The listing builds one solid part. Answer for the finished solid, in the listing's coordinates (mm). Face numbers are marked on the shaded views. A direction names the side the tool comes from. Coordinates: 2 decimals unless noted, no trailing zeros. Order: outer loops, then holes, each group sorted by start corner. A loop starts at its lowest first (then second) coordinate and runs counter-clockwise, first axis right, second up. Notation, with made-up numbers: (-21.5, 42.5) -> (37.5, 42.5) arc R27 ccw to (37.5, 61.5) -> close; hole circle Ø1 at (88.25, -29.75). An arc over 180 degrees is marked (long way). Return JSON: item names as keys, results as strings.
```python
from build123d import *

# Parameters (mm, degrees)
SKETCH_1_W          = 28
SKETCH_1_H          = 16
SKETCH_1_R          = 1.5
EXTRUDE_1_DEPTH     = 10
FILLET_1_R          = 3
SKETCH_2_R          = 1.5
EXTRUDE_2_DEPTH     = 0.4
CUT_EXTRUDE_1_DEPTH = 0.1
CUT_EXTRUDE_2_DEPTH = 3
CUT_EXTRUDE_3_DEPTH = 0.1
CUT_EXTRUDE_4_DEPTH = 0.1
SKETCH_7_W          = 2.9
SKETCH_7_H          = 0.1
CUT_EXTRUDE_5_DEPTH = 0.1
SKETCH_8_W          = 2.9
SKETCH_8_H          = 0.1
CUT_EXTRUDE_6_DEPTH = 0.1
EXTRUDE_3_DEPTH     = 4.5
SKETCH_11_W         = 10
SKETCH_11_H         = 0.8
EXTRUDE_4_DEPTH     = 6.5
SKETCH_12_R         = 0.75
CUT_EXTRUDE_7_DEPTH = 53.388166603
FILLET_2_R          = 1
SKETCH_13_R         = 0.75
CUT_EXTRUDE_8_DEPTH = 2


with BuildPart() as part:
    # Sketch 1 → Extrude 1 (new body)
    with BuildSketch(Plane(origin=(0, 0, 0), x_dir=(0, 0, -1), z_dir=(1, 0, 0))):
        Rectangle(SKETCH_1_W, SKETCH_1_H)
        with Locations((11, -5)):
            Circle(SKETCH_1_R, mode=Mode.SUBTRACT)
        with Locations((-11, 5)):
            Circle(SKETCH_1_R, mode=Mode.SUBTRACT)
    extrude(amount=EXTRUDE_1_DEPTH)

    # Fillet 1
    fillet_1_edges = [part.edges().sort_by_distance(p)[0] for p in [
        (5, 8, 14),
        (5, 8, -14),
        (5, -8, -14),
        (5, -8, 14),
    ]]
    fillet(fillet_1_edges, radius=FILLET_1_R)

    # Sketch 2 → Extrude 2 (add)
    # profile 1 of 2: a face of its own
    with BuildSketch(Plane(origin=(10, 0, 0), x_dir=(0, 0, -1), z_dir=(1, 0, 0))):
        with BuildLine():
            Line((13.5, -5), (13.5, -2.1))
            Line((13.5, -2.1), (11, -2.1))
            ThreePointArc((11, -2.1), (8.949390335, -2.949390335), (8.1, -5))
            Line((8.1, -5), (8.1, -7.5))
            Line((8.1, -7.5), (11, -7.5))
            ThreePointArc((11, -7.5), (12.767766953, -6.767766953), (13.5, -5))
        make_face()
        with Locations((11, -5)):
            Circle(SKETCH_2_R, mode=Mode.SUBTRACT)
    # profile 2 of 2: a face of its own
    with BuildSketch(Plane(origin=(10, 0, 0), x_dir=(0, 0, -1), z_dir=(1, 0, 0))):
        with BuildLine():
            Line((-11, 2.1), (-13.5, 2.1))
            Line((-13.5, 2.1), (-13.5, 5))
            ThreePointArc((-13.5, 5), (-12.767766953, 6.767766953), (-11, 7.5))
            Line((-11, 7.5), (-8.1, 7.5))
            Line((-8.1, 7.5), (-8.1, 5))
            ThreePointArc((-8.1, 5), (-8.949390335, 2.949390335), (-11, 2.1))
        make_face()
        with Locations((-11, 5)):
            Circle(SKETCH_2_R, mode=Mode.SUBTRACT)
    extrude(amount=EXTRUDE_2_DEPTH)

    # Sketch 3 → Cut-Extrude 1 (cut)
    with BuildSketch(Plane.ZY):
        with BuildLine():
            Line((-13.5, -2.1), (-11, -2.1))
            ThreePointArc((-11, -2.1), (-8.949390335, -2.949390335), (-8.1, -5))
            Line((-8.1, -5), (-8.1, -7.5))
            Line((-8.1, -7.5), (-8.1, -8))
            Line((-8.1, -8), (-8.2, -8))
            Line((-8.2, -8), (-8.2, -7.5))
            Line((-8.2, -7.5), (-8.2, -5))
            ThreePointArc((-8.2, -5), (-9.020101013, -3.020101013), (-11, -2.2))
            Line((-11, -2.2), (-13.5, -2.2))
            Line((-13.5, -2.2), (-14, -2.2))
            Line((-14, -2.2), (-14, -2.1))
            Line((-14, -2.1), (-13.5, -2.1))
        make_face()
        with BuildLine():
            Line((13.5, 2.1), (11, 2.1))
            ThreePointArc((11, 2.1), (8.949390335, 2.949390335), (8.1, 5))
            Line((8.1, 5), (8.1, 7.5))
            Line((8.1, 7.5), (8.1, 8))
            Line((8.1, 8), (8.2, 8))
            Line((8.2, 8), (8.2, 7.5))
            Line((8.2, 7.5), (8.2, 5))
            ThreePointArc((8.2, 5), (9.020101013, 3.020101013), (11, 2.2))
            Line((11, 2.2), (13.5, 2.2))
            Line((13.5, 2.2), (14, 2.2))
            Line((14, 2.2), (14, 2.1))
            Line((14, 2.1), (13.5, 2.1))
        make_face()
    extrude(amount=-CUT_EXTRUDE_1_DEPTH, mode=Mode.SUBTRACT)

    # Sketch 4 → Cut-Extrude 2 (cut)
    with BuildSketch(Plane(origin=(0, 8, 0), x_dir=(1, 0, 0), z_dir=(0, 1, 0))):
        Polygon((0, -8.2), (3.1, -8.2), (3.1, 14), (3, 14), (3, -8.1), (0, -8.1), align=None)
    extrude(amount=-CUT_EXTRUDE_2_DEPTH, mode=Mode.SUBTRACT)

    # Sketch 5 → Cut-Extrude 3 (cut)
    with BuildSketch(Plane(origin=(0, 0, -14), x_dir=(-1, 0, 0), z_dir=(0, 0, -1))):
        Polygon((-3, 5), (-3, -2.1), (-0.1, -2.1), (-0.1, -2.2), (-3.1, -2.2), (-3.1, 5), align=None)
    extrude(amount=-CUT_EXTRUDE_3_DEPTH, mode=Mode.SUBTRACT)

    # Sketch 6 → Cut-Extrude 4 (cut)
    with BuildSketch(Plane.ZY.offset(-3.1)):
        with BuildLine():
            Line((-8.2, -8), (11, -8))
            ThreePointArc((11, -8), (13.121320344, -7.121320344), (14, -5))
            Line((14, -5), (14, 2.1))
            Line((14, 2.1), (14, 2.2))
            Line((14, 2.2), (13.9, 2.2))
            Line((13.9, 2.2), (13.9, 2.1))
            Line((13.9, 2.1), (13.9, -5))
            ThreePointArc((13.9, -5), (13.050609665, -7.050609665), (11, -7.9))
            Line((11, -7.9), (-8.2, -7.9))
            Line((-8.2, -7.9), (-8.2, -8))
        make_face()
    extrude(amount=CUT_EXTRUDE_4_DEPTH, mode=Mode.SUBTRACT)

    # Sketch 7 → Cut-Extrude 5 (cut)
    with BuildSketch(Plane.XY.offset(14)):
        with Locations((1.55, 2.15)):
            Rectangle(SKETCH_7_W, SKETCH_7_H)
    extrude(amount=-CUT_EXTRUDE_5_DEPTH, mode=Mode.SUBTRACT)

    # Sketch 8 → Cut-Extrude 6 (cut)
    with BuildSketch(Plane.XZ.offset(8)):
        with Locations((1.55, -8.15)):
            Rectangle(SKETCH_8_W, SKETCH_8_H)
    extrude(amount=-CUT_EXTRUDE_6_DEPTH, mode=Mode.SUBTRACT)

    # Sketch 10 → Extrude 3 (add)
    with BuildSketch(Plane.ZY.offset(-3.1)):
        Polygon((-2.6, -8), (-2.6, -10), (49.4, -10), (49.4, -9.5), (-2.1, -9.5), (-2.1, -8), align=None)
        with BuildLine():
            Line((11, -8.08), (11, -8))
            Line((11, -8), (8.2, -8))
            Line((8.2, -8), (8.2, -8.08))
            ThreePointArc((8.2, -8.08), (9.6, -9.48), (11, -8.08))
        make_face()
    extrude(amount=-EXTRUDE_3_DEPTH)

    # Sketch 11 → Extrude 4 (add)
    with BuildSketch(Plane.ZY.offset(-2)):
        with Locations((-19, 3.6)):
            Rectangle(SKETCH_11_W, SKETCH_11_H)
        with Locations((-19, -2.2)):
            Rectangle(SKETCH_11_W, SKETCH_11_H)
        Polygon((-1, 8), (-1, 10.5), (-10.5, 10.5), (-10.5, 9.7), (-1.8, 9.7), (-1.8, 8), align=None)
    extrude(amount=-EXTRUDE_4_DEPTH)

    # Sketch 12 → Cut-Extrude 7 (cut, through all)
    with BuildSketch(Plane(origin=(0, 4, 0), x_dir=(1, 0, 0), z_dir=(0, 1, 0))):
        with Locations(Location((5.25, 20, 0), (0, 0, 270))):
            Circle(SKETCH_12_R)
        Polygon((2, 17.5), (3, 17.5), (3, 22), (4.154700538, 24), (3, 24), (2, 24), align=None)
        Polygon((8.5, 24), (8.5, 17.5), (7.5, 17.5), (7.5, 22), (6.345299462, 24), (7.5, 24), align=None)
    extrude(amount=-CUT_EXTRUDE_7_DEPTH, mode=Mode.SUBTRACT)

    # Fillet 2
    fillet_2_edges = [part.edges().sort_by_distance(p)[0] for p in [
        (5.35, -10, -2.6),
        (5.35, -9.5, -2.1),
        (5.25, 9.7, -1.8),
        (5.25, 10.5, -1),
    ]]
    fillet(fillet_2_edges, radius=FILLET_2_R)

    # Sketch 13 → Cut-Extrude 8 (cut)
    with BuildSketch(Plane(origin=(0, 10.5, 0), x_dir=(1, 0, 0), z_dir=(0, 1, 0))):
        with Locations(Location((5.25, 6.5, 0), (0, 0, 270))):
            Circle(SKETCH_13_R)
        Polygon((8.5, 10.5), (6.345299462, 10.5), (7.5, 8.5), (7.5, 4), (8.5, 4), align=None)
        Polygon((3, 4), (2, 4), (2, 10.5), (4.154700538, 10.5), (3, 8.5), align=None)
    extrude(amount=-CUT_EXTRUDE_8_DEPTH, mode=Mode.SUBTRACT)


solid = part.part
```
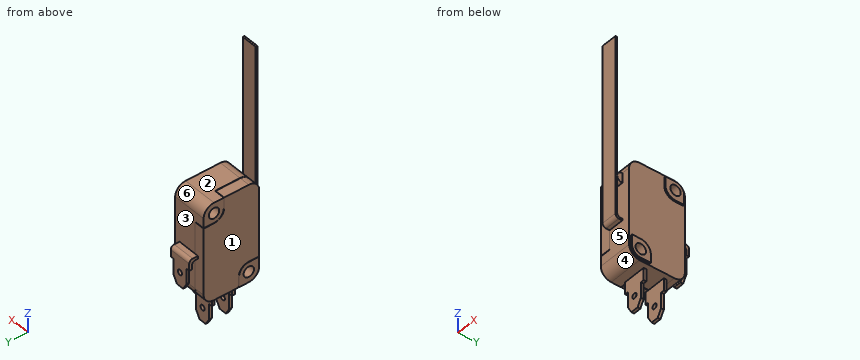
Item 1: Which of the six approach directions +Z, -Z, +X, -X, +Y, -Y give full straight-line access (tool end or side, diameter ignored) to the marked faces 1 and 2?
Answer list:
{"face 1": "+Z, -Z, -X, +Y, -Y", "face 2": "+Z, +X, -X, +Y"}
Item 2: Determine the mould class of the marked faces 3, 4, 5 and 6 for opening direction Y: pulls with the +Y half, pulls with the -Y half, needs draft (parallel to the pull), parting line crosses it, or undercut.
Answer list:
{"face 3": "undercut", "face 4": "pulls with the -Y half", "face 5": "undercut", "face 6": "pulls with the +Y half"}
Item 3: Find the intervals of material crossed by probe 1 along X at (y, z) = (3.55, -20); probe 2 along Y at (x, z) = (9.75, -11); probe 3 along Y at (x, z) = (5.25, 16.5), in increasing order.
Answer list:
{"probe 1": "3 to 4.5, 6 to 7.5", "probe 2": "-8 to -6.5, -3.5 to 8", "probe 3": "-10 to -9.5"}
Item 4: Flat-ended cylindrical pins translate along their axes: pin 1 (1.7 mm diameter, centred on x = 5.25, z = -20, fed in from +Y); pin 2 (0.9 mm diameter, centred on y = 4, z = -20.5, fed in from +X); pin 3 (3 mm diameter, centred on x = 6.5, y = 1, fed in from +Z). Find the tip coordinate at first contact, or state that the pin passes through.
Answer list:
{"pin 1": "y = 4", "pin 2": "x = 7.5", "pin 3": "z = 14"}
Item 5: The part is cut by section B-B on z = 4.5. Determine the outline of the cut face in (x, y), plus the area to 3 significant figures.
Answer list:
{"outline": "(0, -8) -> (3, -8) -> (3, -7.9) -> (3.1, -7.9) -> (3.1, -8) -> (10, -8) -> (10, 8) -> (3.1, 8) -> (3.1, 5) -> (3, 5) -> (3, 8) -> (0, 8) -> close; (3.1, -10) -> (7.6, -10) -> (7.6, -9.5) -> (3.1, -9.5) -> close", "area": "162 mm2"}
Item 6: The part is cut by section A-A on z = -6.5. Determine the outline of the cut face in (x, y).
Answer list:
{"outline": "(0, -8) -> (3, -8) -> (3, -7.9) -> (3.1, -7.9) -> (3.1, -8) -> (10, -8) -> (10, 8) -> (3.1, 8) -> (3.1, 5) -> (3, 5) -> (3, 8) -> (0, 8) -> close; (3, 9.7) -> (4.5, 9.7) -> (4.5, 10.5) -> (3, 10.5) -> close; (6, 9.7) -> (7.5, 9.7) -> (7.5, 10.5) -> (6, 10.5) -> close"}
Item 7: The part is cut by section D-D on z = 34. Determine the outline of the cut face in (x, y), plus the area to 3 significant figures.
Answer list:
{"outline": "(3.1, -10) -> (7.6, -10) -> (7.6, -9.5) -> (3.1, -9.5) -> close", "area": "2.25 mm2"}
Item 8: The part is cut by section C-C on z = -20. Determine the outline of the cut face in (x, y).
Answer list:
{"outline": "(3, -2.6) -> (4.5, -2.6) -> (4.5, -1.8) -> (3, -1.8) -> close; (3, 3.2) -> (4.5, 3.2) -> (4.5, 4) -> (3, 4) -> close; (6, -2.6) -> (7.5, -2.6) -> (7.5, -1.8) -> (6, -1.8) -> close; (6, 3.2) -> (7.5, 3.2) -> (7.5, 4) -> (6, 4) -> close"}
